The listing builds one solid part. Answer for the finished solid, in the listing's coordinates (mm). A direction names the side the tool comes from. Coordinates: 2 decimals unless noted, no trailing zeros. Order: outer loops, then holes, each group sorted by start corner. A loop starts at its lowest first (then second) coordinate and runs counter-clockwise, first axis right, second up. Notation, with made-up numbers: (32, 59) -> (40, 59) arc R20 ccw to (40, 92) -> close; hole circle Ø2 at (7, 65.25). An arc over 180 degrees is marked (long way). One line per question, with ' | ' between items.
from build123d import *

# Parameters (mm, degrees)
SWEEP_THIN1_PROFILE_R   = 145
SWEEP_THIN1_PROFILE_R_2 = 105
BOSS_EXTRUDE2_DEPTH     = 50
SKETCH26_R              = 30
SKETCH26_R_2            = 15
CUT_EXTRUDE2_DEPTH      = 10
SKETCH26_3_R            = 15
CUT_EXTRUDE3_DEPTH      = 50
BOSS_EXTRUDE3_DEPTH     = 50
SKETCH28_R              = 30
SKETCH28_R_2            = 15
CUT_EXTRUDE4_DEPTH      = 10
SKETCH28_3_R            = 15
CUT_EXTRUDE5_DEPTH      = 50
CHAMFER1_SIZE           = 10
SKETCH29_R              = 105
CUT_EXTRUDE7_DEPTH      = 75
CUT_EXTRUDE8_START      = -75
SKETCH30_R              = 105
CUT_EXTRUDE8_DEPTH      = 75
CHAMFER2_SIZE           = 10
CHAMFER3_SIZE           = 10


with BuildPart() as part:
    # Sweep-Thin1: sweep along a path in Sketch1
    with BuildLine(Plane.XY) as sweep_thin1_path:
        Line((0, 410), (0, 260))
        ThreePointArc((0, 260), (76.152236891, 76.152236891), (260, 0))
        Line((260, 0), (410, 0))
    # Sweep-Thin1 profile (on start of the path) → Sweep-Thin1 (sweep)
    with BuildSketch(Plane(origin=(0, 410, 0), x_dir=(0, 0, -1), z_dir=(0, -1, 0))):
        Circle(SWEEP_THIN1_PROFILE_R)
        Circle(SWEEP_THIN1_PROFILE_R_2, mode=Mode.SUBTRACT)
    sweep(path=sweep_thin1_path.line)

    # Sketch24 → Boss-Extrude2 (add)
    with BuildSketch(Plane(origin=(410, 0, 0), x_dir=(0, 0, -1), z_dir=(1, 0, 0))):
        with BuildLine():
            Line((-160, 180), (160, 180))
            ThreePointArc((160, 180), (174.142135624, 174.142135624), (180, 160))
            Line((180, 160), (180, -160))
            ThreePointArc((180, -160), (174.142135624, -174.142135624), (160, -180))
            Line((160, -180), (-160, -180))
            ThreePointArc((-160, -180), (-174.142135624, -174.142135624), (-180, -160))
            Line((-180, -160), (-180, 160))
            ThreePointArc((-180, 160), (-174.142135624, 174.142135624), (-160, 180))
        make_face()
    extrude(amount=BOSS_EXTRUDE2_DEPTH)

    # Sketch26 → Cut-Extrude2 (cut)
    # profile 1 of 4: a face of its own
    with BuildSketch(Plane(origin=(460, 0, 0), x_dir=(0, 0, -1), z_dir=(1, 0, 0))):
        with Locations((-130, 130)):
            Circle(SKETCH26_R)
        with Locations((-130, 130)):
            Circle(SKETCH26_R_2, mode=Mode.SUBTRACT)
    # profile 2 of 4: a face of its own
    with BuildSketch(Plane(origin=(460, 0, 0), x_dir=(0, 0, -1), z_dir=(1, 0, 0))):
        with Locations((-130, -130)):
            Circle(SKETCH26_R)
        with Locations((-130, -130)):
            Circle(SKETCH26_R_2, mode=Mode.SUBTRACT)
    # profile 3 of 4: a face of its own
    with BuildSketch(Plane(origin=(460, 0, 0), x_dir=(0, 0, -1), z_dir=(1, 0, 0))):
        with Locations((130, 130)):
            Circle(SKETCH26_R)
        with Locations((130, 130)):
            Circle(SKETCH26_R_2, mode=Mode.SUBTRACT)
    # profile 4 of 4: a face of its own
    with BuildSketch(Plane(origin=(460, 0, 0), x_dir=(0, 0, -1), z_dir=(1, 0, 0))):
        with Locations((130, -130)):
            Circle(SKETCH26_R)
        with Locations((130, -130)):
            Circle(SKETCH26_R_2, mode=Mode.SUBTRACT)
    extrude(amount=-CUT_EXTRUDE2_DEPTH, mode=Mode.SUBTRACT)

    # Sketch26<3> → Cut-Extrude3 (cut)
    with BuildSketch(Plane(origin=(460, 0, 0), x_dir=(0, 0, -1), z_dir=(1, 0, 0))):
        with Locations((-130, 130)):
            Circle(SKETCH26_3_R)
        with Locations((-130, -130)):
            Circle(SKETCH26_3_R)
        with Locations((130, -130)):
            Circle(SKETCH26_3_R)
        with Locations((130, 130)):
            Circle(SKETCH26_3_R)
    extrude(amount=-CUT_EXTRUDE3_DEPTH, mode=Mode.SUBTRACT)

    # Sketch27 → Boss-Extrude3 (add)
    with BuildSketch(Plane(origin=(0, 410, 0), x_dir=(1, 0, 0), z_dir=(0, 1, 0))):
        with BuildLine():
            Line((-160, 180), (160, 180))
            ThreePointArc((160, 180), (174.142135624, 174.142135624), (180, 160))
            Line((180, 160), (180, -160))
            ThreePointArc((180, -160), (174.142135624, -174.142135624), (160, -180))
            Line((160, -180), (-160, -180))
            ThreePointArc((-160, -180), (-174.142135624, -174.142135624), (-180, -160))
            Line((-180, -160), (-180, 160))
            ThreePointArc((-180, 160), (-174.142135624, 174.142135624), (-160, 180))
        make_face()
    extrude(amount=BOSS_EXTRUDE3_DEPTH)

    # Sketch28 → Cut-Extrude4 (cut)
    # profile 1 of 4: a face of its own
    with BuildSketch(Plane(origin=(0, 460, 0), x_dir=(1, 0, 0), z_dir=(0, 1, 0))):
        with Locations(Location((-130, 130, 0), (0, 0, 270))):
            Circle(SKETCH28_R)
        with Locations(Location((-130, 130, 0), (0, 0, 270))):
            Circle(SKETCH28_R_2, mode=Mode.SUBTRACT)
    # profile 2 of 4: a face of its own
    with BuildSketch(Plane(origin=(0, 460, 0), x_dir=(1, 0, 0), z_dir=(0, 1, 0))):
        with Locations(Location((-130, -130, 0), (0, 0, 270))):
            Circle(SKETCH28_R)
        with Locations(Location((-130, -130, 0), (0, 0, 270))):
            Circle(SKETCH28_R_2, mode=Mode.SUBTRACT)
    # profile 3 of 4: a face of its own
    with BuildSketch(Plane(origin=(0, 460, 0), x_dir=(1, 0, 0), z_dir=(0, 1, 0))):
        with Locations(Location((130, -130, 0), (0, 0, 270))):
            Circle(SKETCH28_R)
        with Locations(Location((130, -130, 0), (0, 0, 270))):
            Circle(SKETCH28_R_2, mode=Mode.SUBTRACT)
    # profile 4 of 4: a face of its own
    with BuildSketch(Plane(origin=(0, 460, 0), x_dir=(1, 0, 0), z_dir=(0, 1, 0))):
        with Locations(Location((130, 130, 0), (0, 0, 270))):
            Circle(SKETCH28_R)
        with Locations(Location((130, 130, 0), (0, 0, 270))):
            Circle(SKETCH28_R_2, mode=Mode.SUBTRACT)
    extrude(amount=-CUT_EXTRUDE4_DEPTH, mode=Mode.SUBTRACT)

    # Sketch28<3> → Cut-Extrude5 (cut)
    with BuildSketch(Plane(origin=(0, 460, 0), x_dir=(1, 0, 0), z_dir=(0, 1, 0))):
        with Locations(Location((-130, 130, 0), (0, 0, 270))):
            Circle(SKETCH28_3_R)
        with Locations(Location((-130, -130, 0), (0, 0, 270))):
            Circle(SKETCH28_3_R)
        with Locations(Location((130, 130, 0), (0, 0, 270))):
            Circle(SKETCH28_3_R)
        with Locations(Location((130, -130, 0), (0, 0, 270))):
            Circle(SKETCH28_3_R)
    extrude(amount=-CUT_EXTRUDE5_DEPTH, mode=Mode.SUBTRACT)

    # Chamfer1
    chamfer1_edges = [part.edges().sort_by_distance(p)[0] for p in [
        (410, 0, 105),
    ]]
    chamfer(chamfer1_edges, length=CHAMFER1_SIZE)

    # Sketch29 → Cut-Extrude7 (cut)
    with BuildSketch(Plane(origin=(460, 0, 0), x_dir=(0, 0, -1), z_dir=(1, 0, 0))):
        Circle(SKETCH29_R)
    extrude(amount=-CUT_EXTRUDE7_DEPTH, mode=Mode.SUBTRACT)

    # Sketch30 → Cut-Extrude8 (cut)
    with BuildSketch(Plane(origin=(0, 460, 0), x_dir=(1, 0, 0), z_dir=(0, 1, 0)).offset(CUT_EXTRUDE8_START)):
        with Locations(Location((0, 0, 0), (0, 0, 180))):
            Circle(SKETCH30_R)
    extrude(amount=CUT_EXTRUDE8_DEPTH, mode=Mode.SUBTRACT)

    # Chamfer2
    chamfer2_edges = [part.edges().sort_by_distance(p)[0] for p in [
        (105, 460, 0),
    ]]
    chamfer(chamfer2_edges, length=CHAMFER2_SIZE)

    # Chamfer3
    chamfer3_edges = [part.edges().sort_by_distance(p)[0] for p in [
        (460, 0, 105),
    ]]
    chamfer(chamfer3_edges, length=CHAMFER3_SIZE)


solid = part.part
Item 1: For faces 1 (the face through (180, 435, -2)), 2 (the face through (43.554, 333.95, -138.304)), 3 (the face through (450, 144, -136)), 4 (the face through (-48.7, 450.6, -93.7)), determine the directions among +Z, -Z, +X, -X, +Y, -Y from which every point of the face is accessible in a straight line to the end or side of a thin tool.
Computed values:
face 1: +Z, -Z, +X, +Y | face 2: none | face 3: +X | face 4: +Y
Item 2: Determine the mould class of faces 5 (the face through (-2, 435, -180)), 6 (the face through (-116, 450, -124)), 7 (the face through (83, 460, -83)), 8 (the face through (140.138, 430.28, 118.944)) for opening direction Z: pulls with the +Z half, pulls with the -Z half, needs draft (parallel to the pull), parting line crosses it, or undercut.
Computed values:
face 5: pulls with the -Z half | face 6: undercut | face 7: needs draft | face 8: undercut
Item 3: Section B-B, the plane z = -128 is taken. Count the separate pieces of the cut face and the enclosed holes in it, plus the area to 3 significant figures.
Computed values:
separate pieces: 5 | enclosed holes: 0 | area: 125,000 mm^2
Item 4: Section A-A, the plane x = 361.5 is taken. Give the vertices of the cut face in (y, z), plus the area to 3 significant figures.
Computed values:
outline: circle Ø290 at (0, 0); hole circle Ø210 at (0, 0) | area: 31,400 mm^2
Item 5: Each of these flat-tipped pins is pushed along its axis until it touches: pin 1 Ø4 at (x, y) = (86, -96) entering from +Z; pin 2 Ø3 at (x, y) = (-76.5, 324) entering from -Z; pin 3 Ø5 at (x, z) = (219.5, -2.5) entering from +Y. Where does it stop, or does it pass through?
Computed values:
pin 1: stops at z = 54.8 | pin 2: stops at z = -124.1 | pin 3: stops at y = 153.32
Item 6: Find the intervals of material crossed by L1, parallel to Y at x = 431.5, z = 130; L2, parallel to Y at x = 378.5, z = 0; L3, parallel to Y at x = -37, z = 152.5, in increasing order.
Computed values:
L1: y = -180 to -145, -115 to 115, 145 to 180 | L2: y = -145 to -105, 105 to 145 | L3: y = 410 to 460
